Part model, mm, in its own coordinate system. Face numbers are marked on the shaded views. Give positions to 0.01 mm unless a question says otherwise; leave off trailing zeros. Order: outer loops, then holes, each group sorted by start corner. A loop starts at its lowest first (then second) coordinate and runs counter-clockwise, first axis right, second up.
1. Slice it at C-C on z = 9.5. Give the number of separate pieces and of enclosed holes in the cut face, and give its area (3 significant figures).
2. Slice it at B-B on y = 89. List the corners of the cut face in (x, z), and give its area (3 significant figures).
3. Drop flat-ended pins along their axis: pin 1 Ø2 at (y, z) = (113.5, 13.5) entering from +X; pin 2 Ø6 at (x, z) = (144, 14.5) entering from -Y; pin 3 Ø10 at (y, z) = (15.5, 13.5) entering from -X. Give the stop position or say it passes through.
4. Mould opens along X. For the marked faces 1, 2 and 3 say: +X half, -X half, draft (parallel to the pull), parting line (faces both ways), or undercut.
5. Probe line 1 (X direction, y = 134, z = 19.25); line 2 (Y direction, x = 72, z = 18); line 3 (X direction, y = 116, z = 3.25). List the from-to ranges inside material, lowest first.
6. Slice it at A-A on x = 26.5. List the corners of the cut face in (y, z), and give its area (3 significant figures).
Solid Edge part; units mm, degrees
sketch "Sketch1" plane through (0, 0, 0) normal (0, 0, 1) x (1, 0, 0)
  line L0 (171, 147) -> (0, 147)
  line L1 (0, 147) -> (0, 0)
  line L2 (0, 0) -> (171, 0)
  line L3 (171, 0) -> (171, 147)
extrude "Protrusion1" add sketch "Sketch1" against normal blind 2
sketch "Sketch2" plane through (0, 0, 0) normal (0, 0, 1) x (1, 0, 0)
  line L0 (113, 74) -> (58, 74)
  line L1 (58, 74) -> (58, 109)
  line L2 (58, 109) -> (113, 109)
  line L3 (113, 109) -> (113, 74)
  line L4 (58, 37) -> (58, 2)
  line L5 (58, 2) -> (113, 2)
  line L6 (113, 2) -> (113, 37)
  line L7 (113, 37) -> (58, 37)
  line L8 (58, 73) -> (58, 38)
  line L9 (58, 38) -> (113, 38)
  line L10 (113, 38) -> (113, 73)
  line L11 (113, 73) -> (58, 73)
  line L12 (2, 73) -> (2, 38)
  line L13 (2, 38) -> (57, 38)
  line L14 (57, 38) -> (57, 73)
  line L15 (57, 73) -> (2, 73)
  line L16 (2, 37) -> (2, 2)
  line L17 (2, 2) -> (57, 2)
  line L18 (57, 2) -> (57, 37)
  line L19 (57, 37) -> (2, 37)
  line L20 (57, 74) -> (2, 74)
  line L21 (2, 74) -> (2, 109)
  line L22 (2, 109) -> (57, 109)
  line L23 (57, 109) -> (57, 74)
  line L24 (171, 147) -> (0, 147)
  line L25 (0, 147) -> (0, 0)
  line L26 (0, 0) -> (171, 0)
  line L27 (171, 0) -> (171, 147)
  line L28 (57, 110) -> (2, 110)
  line L29 (2, 110) -> (2, 145)
  line L30 (2, 145) -> (57, 145)
  line L31 (57, 145) -> (57, 110)
  line L32 (114, 73) -> (169, 73)
  line L33 (169, 73) -> (169, 38)
  line L34 (169, 38) -> (114, 38)
  line L35 (114, 38) -> (114, 73)
  line L36 (114, 37) -> (169, 37)
  line L37 (169, 37) -> (169, 2)
  line L38 (169, 2) -> (114, 2)
  line L39 (114, 2) -> (114, 37)
  line L40 (113, 145) -> (113, 110)
  line L41 (113, 110) -> (58, 110)
  line L42 (58, 110) -> (58, 145)
  line L43 (58, 145) -> (113, 145)
  line L44 (169, 109) -> (114, 109)
  line L45 (114, 109) -> (114, 74)
  line L46 (114, 74) -> (169, 74)
  line L47 (169, 74) -> (169, 109)
  line L48 (114, 145) -> (114, 110)
  line L49 (114, 110) -> (169, 110)
  line L50 (169, 110) -> (169, 145)
  line L51 (169, 145) -> (114, 145)
extrude "FuseBoxHolder" add sketch "Sketch2" along normal blind 20
sketch "Sketch3" plane through (0, 0, 0) normal (0, 0, 1) x (1, 0, 0)
  line L0 (171.75, -0.75) -> (171.75, 147.75)
  line L1 (171.75, 147.75) -> (-0.75, 147.75)
  line L2 (-0.75, 147.75) -> (-0.75, -0.75)
  line L3 (-0.75, -0.75) -> (171.75, -0.75)
extrude "FuseBoxLidGround" add sketch "Sketch3" against normal blind 2
sketch "Sketch4" plane through (0, 0, 0) normal (0, 0, 1) x (1, 0, 0)
  line L0 (-0.25, 147.25) -> (-0.25, -0.25)
  line L1 (-0.25, -0.25) -> (171.25, -0.25)
  line L2 (171.25, -0.25) -> (171.25, 147.25)
  line L3 (171.25, 147.25) -> (-0.25, 147.25)
  line L4 (171.75, -0.75) -> (171.75, 147.75)
  line L5 (171.75, 147.75) -> (-0.75, 147.75)
  line L6 (-0.75, 147.75) -> (-0.75, -0.75)
  line L7 (-0.75, -0.75) -> (171.75, -0.75)
extrude "FuseBoxLidWalls" add sketch "Sketch4" along normal blind 5
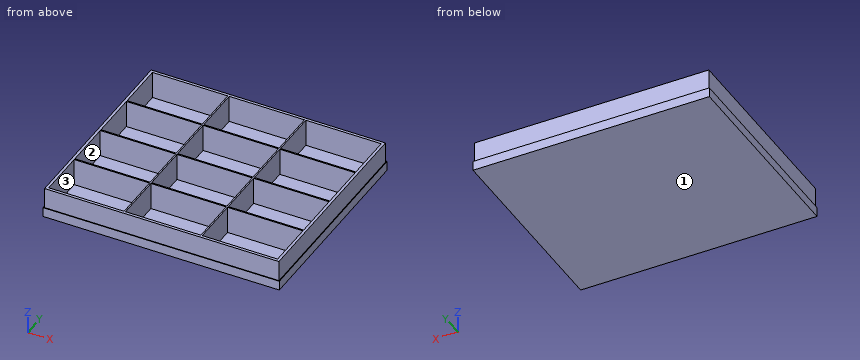
Data:
1. separate pieces: 1
1. enclosed holes: 12
1. area: 2,040 mm2
2. outline: (-0.75, -2) - (171.75, -2) - (171.75, 5) - (171.25, 5) - (171.25, 0) - (171, 0) - (171, 20) - (169, 20) - (169, 0) - (114, 0) - (114, 20) - (113, 20) - (113, 0) - (58, 0) - (58, 20) - (57, 20) - (57, 0) - (2, 0) - (2, 20) - (0, 20) - (0, 0) - (-0.25, 0) - (-0.25, 5) - (-0.75, 5) - close
2. area: 470 mm2
3. pin 1: stops at x = 171
3. pin 2: stops at y = 0
3. pin 3: stops at x = 0
4. face 1: draft
4. face 2: undercut
4. face 3: undercut
5. line 1: x = 0 to 2, 57 to 58, 113 to 114, 169 to 171
5. line 2: y = 0 to 2, 37 to 38, 73 to 74, 109 to 110, 145 to 147
5. line 3: x = -0.75 to -0.25, 0 to 2, 57 to 58, 113 to 114, 169 to 171, 171.25 to 171.75
6. outline: (-0.75, -2) - (147.75, -2) - (147.75, 5) - (147.25, 5) - (147.25, 0) - (147, 0) - (147, 20) - (145, 20) - (145, 0) - (110, 0) - (110, 20) - (109, 20) - (109, 0) - (74, 0) - (74, 20) - (73, 20) - (73, 0) - (38, 0) - (38, 20) - (37, 20) - (37, 0) - (2, 0) - (2, 20) - (0, 20) - (0, 0) - (-0.25, 0) - (-0.25, 5) - (-0.75, 5) - close
6. area: 442 mm2
